Design review of the part built by this model. Coordinates are the model's own, in mm. Face numbers are marked on the shaded views. A direction names the side the tool comes from. Coordinates: 2 decimals unless noted, no trailing zeros. Loops run counter-clockwise (first coordinate to the right, second up) from the corner with the lowest first, then second, coordinate; pieces in that order, holes last. Notation, with made-up numbers: (80, -8) -> (139, -8) arc R30 cw to (139, 28) -> close; hole circle Ø11 at (51, -3.75). An arc over 180 degrees is marked (long way). Use one line per item in the form item = value. Start each with the question number.
1. Consider section B-B (x = -15.5). State the section outline as (y, z) points, then the cut area to 3 significant figures.
2. Consider section D-D (z = 3.5). State the section outline as (x, y) points, then the cut area to 3 significant figures.
3. Consider section A-A (z = 1). State the section outline as (x, y) points.
4. Consider section C-C (z = 10.5). State the section outline as (x, y) points, then the cut area to 3 significant figures.
5. Wall thickness on line 1 (X direction, y = -6.5, z = 11.5); line 2 (Y direction, x = -7.5, z = 9.25); line 3 (X direction, y = 0, z = 1.25): over which ranges is each line inside the solid? List them lowest first. Write a range as from..to.
6. Machinability: for the marked faces 1, 2 and 3, which of the approach directions +Z, -Z, +X, -X, +Y, -Y give a long, thin tool a straight path to every point of the face, cutting with its end or side? Answer none if there is none.
7. For pin 1 (6 mm diameter, centred on y = 3, z = 10.5, fed in from +X); pin 2 (7.5 mm diameter, centred on x = -16, y = 4, fed in from +Z); pin 3 (3.5 mm diameter, centred on y = 0, z = 8.5, fed in from -X), all flat-tipped, find the tip position at first contact; note any pin that passes through.
Autodesk Inventor part; units mm, degrees
ref_plane "YZ Plane" through (0, 0, 0) normal (1, 0, 0) x (0, 1, 0)
ref_plane "XZ Plane" through (0, 0, 0) normal (0, 1, 0) x (-1, 0, 0)
ref_plane "XY Plane" through (0, 0, 0) normal (0, 0, 1) x (1, 0, 0)
sketch "Sketch1" plane through (0, 0, 0) normal (0, 0, 1) x (1, 0, 0)
  line L0 (-19, -12.5) -> (19, -12.5)
  line L1 (19, -12.5) -> (19, 12.5)
  line L2 (19, 12.5) -> (-19, 12.5)
  line L3 (-19, 12.5) -> (-19, -12.5)
  line L4 (-19, -12.5) -> (19, 12.5) construction
  line L5 (19, -12.5) -> (-19, 12.5) construction
  point P0 (0, 0)
  dimension "d0" = 38
  dimension "d1" = 25
extrude "Extrusion1" add sketch "Sketch1" along normal blind 2
sketch "Sketch2" plane through (0, 0, 2) normal (0, 0, 1) x (1, 0, 0)
  line L0 (19, 12.5) -> (-19, 12.5)
  line L1 (-12, -12.5) -> (12, -12.5)
  line L2 (12, -12.5) -> (12, 12.5)
  line L3 (12, 12.5) -> (-12, 12.5)
  line L4 (-12, 12.5) -> (-12, -12.5)
  line L5 (-12, -12.5) -> (12, 12.5) construction
  line L6 (12, -12.5) -> (-12, 12.5) construction
  point P0 (0, 0)
  dimension "d4" = 24
extrude "Extrusion2" add sketch "Sketch2" along normal blind 12
sketch "Sketch3" plane through (0, 0, 2) normal (0, 0, 1) x (1, 0, 0)
  line L0 (-15, 0) -> (15, 0) construction
  point P0 (0, 0)
  point P1 (0, 0)
  dimension "d7" = 30
hole "Hole1" at (-15, 0, 2) at (15, 0, 2) direction (0, 0, -1) diameter 4 end through all
sketch "Sketch4" plane through (0, 0, 14) normal (0, 0, 1) x (1, 0, 0)
  line L0 (-7.5, -6.5) -> (7.5, -6.5) construction
  line L1 (7.5, -6.5) -> (7.5, 6.5) construction
  line L2 (7.5, 6.5) -> (-7.5, 6.5) construction
  line L3 (-7.5, 6.5) -> (-7.5, -6.5) construction
  line L4 (-7.5, -6.5) -> (7.5, 6.5) construction
  line L5 (7.5, -6.5) -> (-7.5, 6.5) construction
  point P0 (0, 0)
  dimension "d15" = 15
  dimension "d16" = 13
hole "Hole2" at (-7.5, 6.5, 14) at (7.5, 6.5, 14) at (7.5, -6.5, 14) at (-7.5, -6.5, 14) direction (0, 0, -1) diameter 3.242 depth 8 tip angle 118
fillet "Fillet1" radius 2 4 edges at (-19, -12.5, 1) (19, -12.5, 1) (19, 12.5, 1) (-19, 12.5, 1)
properties part number "GT175DA120U"
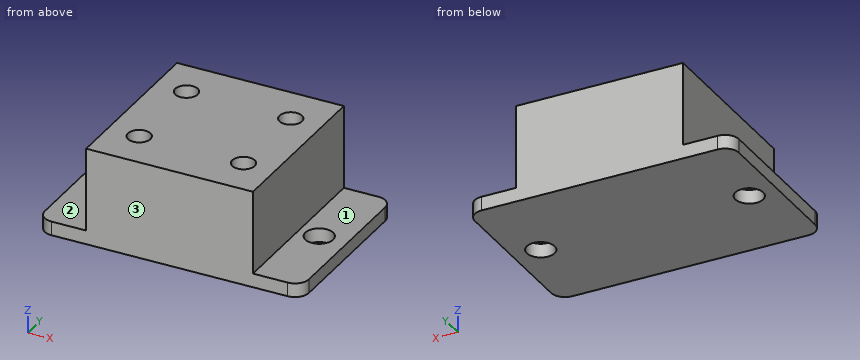
Geometry check:
q1.outline = (-12.5, 0) -> (-1.94, 0) -> (-1.94, 2) -> (-12.5, 2) -> close; (1.94, 0) -> (12.5, 0) -> (12.5, 2) -> (1.94, 2) -> close
q1.area = 42.3 mm²
q2.outline = (-12, -12.5) -> (12, -12.5) -> (12, 12.5) -> (-12, 12.5) -> close
q2.area = 600 mm²
q3.outline = (-19, -10.5) arc R2 ccw to (-17, -12.5) -> (17, -12.5) arc R2 ccw to (19, -10.5) -> (19, 10.5) arc R2 ccw to (17, 12.5) -> (-17, 12.5) arc R2 ccw to (-19, 10.5) -> close; hole circle Ø4 at (-15, 0); hole circle Ø4 at (15, 0)
q4.outline = (-12, -12.5) -> (12, -12.5) -> (12, 12.5) -> (-12, 12.5) -> close; hole circle Ø3.24 at (-7.5, -6.5); hole circle Ø3.24 at (-7.5, 6.5); hole circle Ø3.24 at (7.5, -6.5); hole circle Ø3.24 at (7.5, 6.5)
q4.area = 567 mm²
q5.line_1 = -12..-9.12, -5.88..5.88, 9.12..12
q5.line_2 = -12.5..-8.12, -4.88..4.88, 8.12..12.5
q5.line_3 = -19..-17, -13..13, 17..19
q6.face_1 = +Z, +X, +Y, -Y
q6.face_2 = +Z, -X, +Y, -Y
q6.face_3 = +Z, -Z, +X, -X, -Y
q7.pin_1 = 12
q7.pin_2 = 2
q7.pin_3 = -12
